The listing builds one solid part. Answer for the finished solid, in the listing's coordinates (mm). A direction names the side the tool comes from. Round coordinates to 2 decimals unless told otherwise and drop trailing zeros. Order: outer loops, then holes, each group sorted by start corner. A loop starts at its lowest first (then second) coordinate and runs counter-clockwise, first axis right, second up. Notation, with made-up numbers: (52.25, 68) -> (83.25, 68) arc R19 cw to (83.25, 73) -> close; hole circle Ø8 at (50, 75.25). An arc over 180 degrees is marked (long way). Answer in a Markdown table with one row per item. Add a question column.
```python
from build123d import *

# Parameters (mm, degrees)
F0_R     = 3.35
F0_R_2   = 2.25
F1_DEPTH = 6.5
F0_R_3   = 6
F2_DEPTH = 5
F3_R     = 3.35
F4_DEPTH = 4


with BuildPart() as f1:
    # F0 (on Top) → F1 (new body)
    with BuildSketch(Plane.XY):
        Circle(F0_R)
        Circle(F0_R_2, mode=Mode.SUBTRACT)
    extrude(amount=F1_DEPTH)

    # F0 (on Top) → F2 (join)
    with BuildSketch(Plane.XY):
        Circle(F0_R_3)
        Circle(F0_R, mode=Mode.SUBTRACT)
    extrude(amount=F2_DEPTH)

    # F3 (on face) + F0 (on Top) → F4 (cut)
    with BuildSketch(Plane.XY):
        Polygon((3.8, 2.193931), (0, 4.387862), (-3.8, 2.193931), (-3.8, -2.193931), (0, -4.387862), (3.8, -2.193931), align=None)
        Circle(F3_R, mode=Mode.SUBTRACT)
    with BuildSketch(Plane.XY):
        Circle(F0_R)
        Circle(F0_R_2, mode=Mode.SUBTRACT)
    extrude(amount=F4_DEPTH, mode=Mode.SUBTRACT)


solid = f1.part
```
Item 1: The part is cut by section C-C, the plane x = 1.25. Give the vertices of the cut face in (y, z).
Item 2: For a pull along X with two mould halves and no side action, classify faces 3 (the face through (1.927, 3.276, 1.972)), 4 (the face through (3, -3, 5)), 5 (the face through (-3.347, 0.147, 5.74)) as released by +X, released by -X, zero draft, split by the parting line, or undercut.
Item 3: Flat-ended cylindrical pins translate along their axes: P1, Ø1.5, axis at y = -4.5, z = 5.5, coming from the +X side; P2, Ø4, axis at x = 0, y = 0, coming from the +Z side. Find the tip coordinate at first contact, or state that the pin passes through.
Item 4: The part is cut by section D-D, the plane x = -3. Give the vertices of the cut face in (y, z).
Item 5: Find the intervals of material crossed by probe 1 along Y at (x, z) = (0, 5.25); probe 2 along Y at (x, z) = (0, 4.5); probe 3 along Z at (x, y) = (3.25, -3.5), in increasing order. Write a range as [from, to].
Item 6: A tool of negligible diameter and unlimited length cuts with its end or side. For faces 1 (the face through (-0.29, 2.23, 5.23)), 2 (the face through (-2, -2, 4)), from which of +Z, -Z, +X, -X, +Y, -Y can it reach the whole face along a straight path? Write none if from no direction.
Item 7: The part is cut by section B-B, the plane z = 3.5. Give the vertices of the cut face in (x, y), and give its area (3 significant figures).
Item 8: The part is cut by section A-A, the plane y = 0. Give the vertices of the cut face in (x, z).
Resolved:
| question | item | result |
|---|---|---|
| 1 | outline | (-5.87, 0) -> (-3.67, 0) -> (-3.67, 4) -> (-1.87, 4) -> (-1.87, 6.5) -> (-3.11, 6.5) -> (-3.11, 5) -> (-5.87, 5) -> close; (1.87, 4) -> (3.67, 4) -> (3.67, 0) -> (5.87, 0) -> (5.87, 5) -> (3.11, 5) -> (3.11, 6.5) -> (1.87, 6.5) -> close |
| 2 | face 3 | undercut |
| 2 | face 4 | zero draft |
| 2 | face 5 | split by the parting line |
| 3 | P1 | x = 4.52 |
| 3 | P2 | through |
| 4 | outline | (-5.2, 0) -> (-2.66, 0) -> (-2.66, 4) -> (2.66, 4) -> (2.66, 0) -> (5.2, 0) -> (5.2, 5) -> (1.49, 5) -> (1.49, 6.5) -> (-1.49, 6.5) -> (-1.49, 5) -> (-5.2, 5) -> close |
| 5 | probe 1 | [-3.35, -2.25], [2.25, 3.35] |
| 5 | probe 2 | [-6, -2.25], [2.25, 6] |
| 5 | probe 3 | [0, 5] |
| 6 | face 1 | +Z, -Z |
| 6 | face 2 | -Z |
| 7 | outline | circle Ø12 at (0, 0); hole (-3.8, -2.19) -> (0, -4.39) -> (3.8, -2.19) -> (3.8, 2.19) -> (0, 4.39) -> (-3.8, 2.19) -> close |
| 7 | area | 63.1 mm2 |
| 8 | outline | (-6, 0) -> (-3.8, 0) -> (-3.8, 4) -> (-2.25, 4) -> (-2.25, 6.5) -> (-3.35, 6.5) -> (-3.35, 5) -> (-6, 5) -> close; (2.25, 4) -> (3.8, 4) -> (3.8, 0) -> (6, 0) -> (6, 5) -> (3.35, 5) -> (3.35, 6.5) -> (2.25, 6.5) -> close |
